from build123d import *

# Parameters (mm, degrees)
F0_W     = 50
F0_H     = 35
F1_DEPTH = 20
F2_R     = 14
F3_DEPTH = 7
F4_R     = 14
F5_DEPTH = 7
F6_R     = 13
F7_DEPTH = 13.001
F8_R     = 3
F9_DEPTH = 25


with BuildPart() as f1:
    # F0 (on Front) → F1 (new body)
    with BuildSketch(Plane.XZ):
        with Locations((25, 17.5)):
            Rectangle(F0_W, F0_H)
    extrude(amount=F1_DEPTH)

    # F2 (on face) → F3 (cut)
    with BuildSketch(Plane.XZ.offset(20)):
        with Locations((25, 15)):
            Circle(F2_R)
    extrude(amount=-F3_DEPTH, mode=Mode.SUBTRACT)

    # F4 (on face) → F5 (cut)
    with BuildSketch(Plane(origin=(0, 0, 0), x_dir=(-1, 0, 0), z_dir=(0, 1, 0))):
        with Locations((-25, 15)):
            Circle(F4_R)
    extrude(amount=-F5_DEPTH, mode=Mode.SUBTRACT)

    # F6 (on face) → F7 (cut, through all)
    with BuildSketch(Plane(origin=(0, -7, 0), x_dir=(-1, 0, 0), z_dir=(0, 1, 0))):
        with Locations((-25, 15)):
            Circle(F6_R)
    extrude(amount=-F7_DEPTH, mode=Mode.SUBTRACT)

    # F8 (on face) → F9 (cut)
    with BuildSketch(Plane(origin=(0, 0, 0), x_dir=(1, 0, 0), z_dir=(0, 0, -1))):
        with Locations((7.5, 10)):
            Circle(F8_R)
        with Locations((42.5, 10)):
            Circle(F8_R)
    extrude(amount=-F9_DEPTH, mode=Mode.SUBTRACT)


solid = f1.part
Read the model definition and answer for the solid it produces. Units are mm, in the model's axes. A direction names the side the tool comes from. Coordinates: 2 decimals unless noted, no trailing zeros. Loops run counter-clockwise (first coordinate to the right, second up) from the corner with the lowest first, then second, coordinate; pieces in that order, holes last.
Q1. The part is cut by section D-D on z = 5.5. Write down the section's boundary in (x, y), and give its area (3 significant figures).
Q2. Each of these flat-tipped pins is pushed along its axis until it touches: pin 1 Ø6 at (y, z) = (-13, 31.5) entering from -X; pin 2 Ø6 at (x, z) = (18, 18.5) entering from -Y. Where does it stop, or does it pass through?
Q3. Consider probe 1 along Z at (x, y) = (25, -8.2); probe 2 along Z at (x, y) = (25, -14.5); probe 3 along Y at (x, z) = (42.5, 15.25). Determine where each line is inside the solid, lowest interval first.
Q4. The part is cut by section B-B on x = 25. Write down the section's boundary in (y, z), and give its area (3 significant figures).
Q5. The part is cut by section C-C on y = -10. Write down the section's boundary in (x, z).
Q6. The part is cut by section A-A on z = 15. Write down the section's boundary in (x, y).
Q7. Which of the six approach directions +Z, -Z, +X, -X, +Y, -Y give full straight-line access (tool end or side, diameter ignored) to faces 4 (the face through (34.3, -13, 5.7)), 5 (the face through (10.27, -8.85, 12.32)), 6 (the face through (24.7, -20, 29.4)), 7 (the face through (28.03, -3.45, 1.33))?
Q8. The mould has two halves that part along Y. Classify faces 1 (the face through (31.5, -16.5, 2.6)), 2 (the face through (7, -10, 25)), 3 (the face through (24.7, 0, 29.4)): +Y half, -Y half, draft (parallel to the pull), parting line (faces both ways), or undercut.
Results below:
1. outline: (0, -20) - (14.72, -20) - (14.72, -13) - (16.13, -13) - (16.13, -7) - (14.72, -7) - (14.72, 0) - (0, 0) - close; (33.87, -13) - (35.28, -13) - (35.28, -20) - (50, -20) - (50, 0) - (35.28, 0) - (35.28, -7) - (33.87, -7) - close; hole circle Ø6 at (7.5, -10); hole circle Ø6 at (42.5, -10)
1. area: 549 mm2
2. pin 1: stops at x = 0
2. pin 2: passes through
3. probe 1: z = 0 to 2, 28 to 35
3. probe 2: z = 0 to 1, 29 to 35
3. probe 3: y = -20 to -13, -7 to 0
4. outline: (-20, 0) - (0, 0) - (0, 1) - (-7, 1) - (-7, 2) - (-13, 2) - (-13, 1) - (-20, 1) - close; (-20, 29) - (-13, 29) - (-13, 28) - (-7, 28) - (-7, 29) - (0, 29) - (0, 35) - (-20, 35) - close
4. area: 152 mm2
5. outline: (0, 0) - (4.5, 0) - (4.5, 25) - (10.5, 25) - (10.5, 0) - (39.5, 0) - (39.5, 25) - (45.5, 25) - (45.5, 0) - (50, 0) - (50, 35) - (0, 35) - close; hole circle Ø26 at (25, 15)
6. outline: (0, -20) - (11, -20) - (11, -13) - (12, -13) - (12, -7) - (11, -7) - (11, 0) - (0, 0) - close; (38, -13) - (39, -13) - (39, -20) - (50, -20) - (50, 0) - (39, 0) - (39, -7) - (38, -7) - close; hole circle Ø6 at (7.5, -10); hole circle Ø6 at (42.5, -10)
7. face 4: -Y
7. face 5: -Z
7. face 6: +Z, -Z, +X, -X, -Y
7. face 7: +Y
8. face 1: draft
8. face 2: undercut
8. face 3: +Y half
